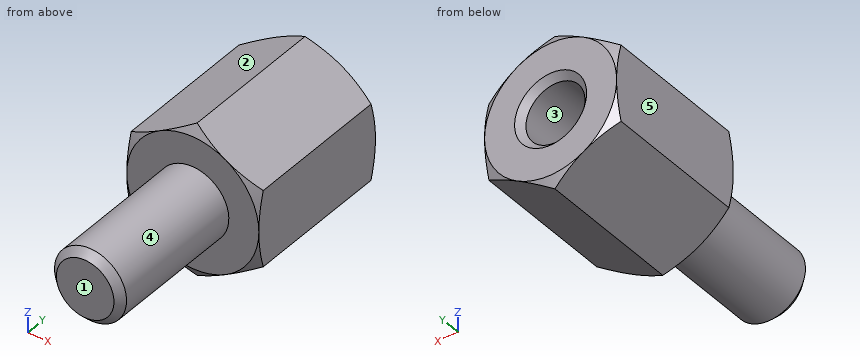
Autodesk Inventor part; units mm, degrees
ref_plane "YZ Plane" through (0, 0, 0) normal (1, 0, 0) x (0, 1, 0)
ref_plane "XZ Plane" through (0, 0, 0) normal (0, 1, 0) x (-1, 0, 0)
ref_plane "XY Plane" through (0, 0, 0) normal (0, 0, 1) x (1, 0, 0)
sketch "スケッチ1" plane through (0, 0, 0) normal (1, 0, 0) x (0, 1, 0)
  line L0 (-3.25, 0) -> (3.25, 0)
  line L1 (0, 0) -> (0, 3.1754) construction
  line L2 (-3.0044, 3.1754) -> (-3.25, 2.75)
  line L3 (-3.25, 2.75) -> (-3.25, 0)
  line L4 (-3.0044, 3.1754) -> (3.0044, 3.1754)
  line L5 (3.0044, 3.1754) -> (3.25, 2.75)
  line L6 (3.25, 2.75) -> (3.25, 0)
  line L7 (-3.25, 1.5) -> (-8.95, 1.5)
  line L8 (-9.25, 1.2) -> (-9.25, 0)
  line L9 (-9.25, 0) -> (-3.25, 0)
  line L10 (-8.95, 1.5) -> (-9.25, 1.2)
  point P0 (3.25, 1.5)
  point P1 (-9.25, 1.5)
  dimension "d1" = 2.75
  dimension "d2" = 3.1754
  dimension "d3" = 30
  dimension "d4" = 6.5
  dimension "d18" = 6
  dimension "d19" = 3
  dimension "d22" = 0.3
  dimension "d23" = 0.3
revolve "回転1" add sketch "スケッチ1" angle 360 about axis through (0, -3.25, 0) along (0, 1, 0)
sketch "スケッチ2" plane through (0, 3.25, 0) normal (0, 1, 0) x (1, 0, 0)
  line L0 (0, -3.1754) -> (-2.75, -1.5877)
  line L1 (-2.75, -1.5877) -> (-2.75, 1.5877)
  line L2 (-2.75, 1.5877) -> (0, 3.1754)
  line L3 (0, 3.1754) -> (2.75, 1.5877)
  line L4 (2.75, 1.5877) -> (2.75, -1.5877)
  line L5 (2.75, -1.5877) -> (0, -3.1754)
  circle A0 centre (0, 0) radius 3.1754
  point P0 (0, 0)
  point P1 (0, 0)
  point P2 (0, 0)
  point P3 (0, 0)
  point P4 (0, 3.1754)
  point P5 (0, 3.1754)
  point P6 (2.75, -1.5877)
  point P7 (2.75, -1.5877)
extrude "押し出し1" cut sketch "スケッチ2" against normal through all contours A0 L0 | L5 A0 | A0 L1 | L4 A0 | A0 L2 | L3 A0
hole "穴1" at (0, 3.25, 0) direction (0, -1, 0) diameter 2.459 depth 3.3 tip angle 118 countersink diameter 3 countersink angle 90
thread "ねじ1"
equation "\"d2\" = 1.1547 * d1"
properties part number "BSL-306.5BE" material "アセタール樹脂、黒"
The model under review builds one solid part; all positions refer to its coordinate system, in mm. Face numbers are marked on the shaded views. A direction names the side the tool comes from. Give positions to 0.01 mm unless a question says otherwise; leave off trailing zeros. Loops run counter-clockwise (first coordinate to the right, second up) from the corner with the lowest first, then second, coordinate; pieces in that order, holes last. Notation, with made-up numbers: (26, 31.25) -> (45, 31.25) arc R23 ccw to (45, 67.25) -> close; hole circle Ø3 at (46.5, 80). An arc over 180 degrees is marked (long way). Answer as a JSON object with one key per item and string values. Group by question number.
Q1. Take a section at B-B (y = -4.5). Write out the cut boundary in (x, z).
Q2. Wall thickness on line 1 along X through (y, z) = (1.2, 0); line 2 along Y through (x, z) = (1.8, 1.5); line 3 along X through (y, z) = (0.5, -0.5): over which ranges is each line inside the solid? List them lowest first.
Q3. Insertion check: pin 1 (2 mm diameter, centred on x = 0, z = 0, fed in from +Y); pin 2 (2 mm diameter, centred on x = -2, y = 2, fed in from -Z). Each pin has a flat end and moves straight along its axis. Give the tip position at first contact, or say it passes through.
Q4. Take a section at A-A (y = -2.75). Write out the cut boundary in (x, z), plus the area to 3 significant figures.
Q5. Tool access review of the marked faces 4 and 5: name each direction out of +Z, -Z, +X, -X, +Y, -Y from which nothing blocks a thin tool from reaching the whole face with its end or side.
Q6. Draft analysis for pull direction Z (two halves, no side actions). For the marked faces 1, 2 and 3, state which applies: pulls with the +Z half, pulls with the -Z half, needs draft (parallel to the pull), parting line crosses it, or undercut.
Answer below:
{
 "1": {"outline": "circle Ø3 at (0, 0)"},
 "2": {"line 1": "x = -2.75 to -1.23, 1.23 to 2.75", "line 2": "y = -3.25 to 3.25", "line 3": "x = -2.75 to -1.12, 1.12 to 2.75"},
 "3": {"pin 1": "stops at y = -0.19", "pin 2": "stops at z = -2.6"},
 "4": {"outline": "(-2.75, -1.59) -> (0, -3.18) -> (2.75, -1.59) -> (2.75, 1.59) -> (0, 3.18) -> (-2.75, 1.59) -> close", "area": "26.2 mm2"},
 "5": {"face 4": "-Y", "face 5": "+Z, -Z, -X, +Y, -Y"},
 "6": {"face 1": "needs draft", "face 2": "pulls with the +Z half", "face 3": "undercut"}
}
